The model under review builds one solid part; all positions refer to its coordinate system, in mm. A direction names the side the tool comes from. Round coordinates to 2 decimals unless told otherwise and drop trailing zeros. Order: outer loops, then holes, each group sorted by start corner. A loop starts at its lowest first (then second) coordinate and runs counter-clockwise, first axis right, second up.
```python
from build123d import *

# Parameters (mm, degrees)
EXTRUDE_1_DEPTH     = 5
SKETCH_3_W          = 5
SKETCH_3_H          = 2
CUT_EXTRUDE_2_DEPTH = 10


with BuildPart() as part:
    # 草图1 → 凸台-拉伸1 (new body)
    with BuildSketch(Plane.XY):
        with BuildLine():
            Line((36.5, -9.5), (36.5, 9.5))
            ThreePointArc((36.5, 9.5), (35.621320344, 11.621320344), (33.5, 12.5))
            Line((33.5, 12.5), (-33.5, 12.5))
            ThreePointArc((-33.5, 12.5), (-35.621320344, 11.621320344), (-36.5, 9.5))
            Line((-36.5, 9.5), (-36.5, -9.5))
            ThreePointArc((-36.5, -9.5), (-35.621320344, -11.621320344), (-33.5, -12.5))
            Line((-33.5, -12.5), (-2.5, -12.5))
            Line((-2.5, -12.5), (-2.5, 2.5))
            Line((-2.5, 2.5), (2.5, 2.5))
            Line((2.5, 2.5), (2.5, -12.5))
            Line((2.5, -12.5), (33.5, -12.5))
            ThreePointArc((33.5, -12.5), (35.621320344, -11.621320344), (36.5, -9.5))
        make_face()
        with BuildLine():
            Line((-19.75, -2.5), (-19.75, 6))
            ThreePointArc((-19.75, 6), (-16.5, 9.25), (-13.25, 6))
            Line((-13.25, 6), (-13.25, -2.5))
            ThreePointArc((-13.25, -2.5), (-16.5, -5.75), (-19.75, -2.5))
        make_face(mode=Mode.SUBTRACT)
        with BuildLine():
            Line((19.75, -2.5), (19.75, 6))
            ThreePointArc((19.75, 6), (16.5, 9.25), (13.25, 6))
            Line((13.25, 6), (13.25, -2.5))
            ThreePointArc((13.25, -2.5), (16.5, -5.75), (19.75, -2.5))
        make_face(mode=Mode.SUBTRACT)
    extrude(amount=EXTRUDE_1_DEPTH)

    # 草图3 → 切除-拉伸2 (cut)
    with BuildSketch(Plane(origin=(0, 0, 0), x_dir=(-1, 0, 0), z_dir=(0, 0, -1))):
        with Locations((0, 3.5)):
            Rectangle(SKETCH_3_W, SKETCH_3_H)
    extrude(amount=-CUT_EXTRUDE_2_DEPTH, mode=Mode.SUBTRACT)


solid = part.part
```
(1) To check wall thickness, follow probe 1 along X at (y, z) = (-2.25, 3.6); probe 2 along X at (y, z) = (-8, 4.35); probe 3 along X at (y, z) = (-4.5, 0.5). State the ranges of each line that lie inside material, in increasing order.
Data:
probe 1: x = -36.5 to -19.75, -13.25 to -2.5, 2.5 to 13.25, 19.75 to 36.5
probe 2: x = -36.5 to -2.5, 2.5 to 36.5
probe 3: x = -36.5 to -19.06, -13.94 to -2.5, 2.5 to 13.94, 19.06 to 36.5
(2) Consider section C-C (y = -8). Write out the cut boundary in (x, z).
Data:
outline: (-36.5, 0) - (-2.5, 0) - (-2.5, 5) - (-36.5, 5) - close; (2.5, 0) - (36.5, 0) - (36.5, 5) - (2.5, 5) - close
(3) Consider section A-A (y = -1.25). Write out the cut boundary in (x, z), and give its area (3 significant figures).
Data:
outline: (-36.5, 0) - (-19.75, 0) - (-19.75, 5) - (-36.5, 5) - close; (-13.25, 0) - (-2.5, 0) - (-2.5, 5) - (-13.25, 5) - close; (2.5, 0) - (13.25, 0) - (13.25, 5) - (2.5, 5) - close; (19.75, 0) - (36.5, 0) - (36.5, 5) - (19.75, 5) - close
area: 275 mm2
(4) For faces 4 (the cylindrical face through (-16.57, 9.25, 2.46)), 5 (the flat face through (2.5, -4, 2)), 6 (the flat face through (36.5, 0, 2)), list the 3-axis set-ups (+Z, -Z, +X, -X, +Y, -Y) from which the entire face can be reached by the end or side of a thin tool; tool diameter is ignored.
Data:
face 4: +Z, -Z
face 5: +Z, -Z, -Y
face 6: +Z, -Z, +X, +Y, -Y
(5) Consider section D-D (x = 16.5). Write out the cut boundary in (y, z), and give its area (3 significant figures).
Data:
outline: (-12.5, 0) - (-5.75, 0) - (-5.75, 5) - (-12.5, 5) - close; (9.25, 0) - (12.5, 0) - (12.5, 5) - (9.25, 5) - close
area: 50.0 mm2
(6) Draft analysis for pull direction X (two halves, no side actions). For faces 1 (the flat face through (0, 4.5, 2)), 2 (the cylindrical face through (35.64, 11.6, 2.46)), 3 (the flat face through (-36.5, 0, 2)), state which applies: pulls with the +X half, pulls with the -X half, needs draft (parallel to the pull), parting line crosses it, or undercut.
Data:
face 1: undercut
face 2: pulls with the +X half
face 3: pulls with the -X half
(7) Consider section B-B (z = 2.6). Write out the cut boundary in (x, y).
Data:
outline: (-36.5, -9.5) arc R3 ccw to (-33.5, -12.5) - (-2.5, -12.5) - (-2.5, 4.5) - (2.5, 4.5) - (2.5, -12.5) - (33.5, -12.5) arc R3 ccw to (36.5, -9.5) - (36.5, 9.5) arc R3 ccw to (33.5, 12.5) - (-33.5, 12.5) arc R3 ccw to (-36.5, 9.5) - close; hole (-19.75, -2.5) arc R3.25 ccw to (-13.25, -2.5) - (-13.25, 6) arc R3.25 ccw to (-19.75, 6) - close; hole (13.25, -2.5) arc R3.25 ccw to (19.75, -2.5) - (19.75, 6) arc R3.25 ccw to (13.25, 6) - close
